Source: CAD feature listing. Evaluate the final solid. Frame: model axes, mm. A direction names the side the tool comes from. Give positions to 0.01 mm unless a question says otherwise; leave off trailing zeros. Answer as a JSON object with one key per item and string values. Group by question number.
Item 1: First-contact query: pin 1 Ø1.4 at (x, z) = (81.5, -1) entering from +Y (3 decimals); pin 2 Ø3.5 at (x, z) = (90.5, -1) entering from -Y; pin 3 Ø2.5 at (x, y) = (59.5, 0.5) entering from -Z (3 decimals). Flat tips, straight axial feed; report the tip coordinate or a pass-through.
Item 2: Ray query, probe 1 along Y at (x, z) = (92.5, -1) (3 decimals); probe 2 along Y at (x, z) = (48.5, -7.25) (3 decimals). Return the intervals inside material, ascending. Write a range as from..to.
Item 3: Pull-direction query (Z, two-part tool) for faces 5 (the face through (74, -7, 10)), 6 (the face through (74, 0, -3.365)), 7 (the face through (74, -8.5, -4)); classes: pulls with the +Z half, pulls with the -Z half, needs draft (parallel to the pull), parting line crosses it, or undercut.
Item 4: Access query for faces 1 (the face through (73.95, -4.18, -5.24)), 2 (the face through (74, -3.365, 0)), 3 (the face through (74, 0, 3.365)), 4 (the face through (74, 10, -7)). Directions: +Z, -Z, +X, -X, +Y, -Y. A direction counts if a zero-diameter tool reaches every point of the face in a straight line with its end or side. Return the directions, or none.
from build123d import *

# Parameters (mm, degrees)
BOSS_EXTRUDE1_DEPTH = 150


with BuildPart() as part:
    # Sketch1 → Boss-Extrude1 (new body)
    with BuildSketch(Plane(origin=(0, 0, 0), x_dir=(0, 0, -1), z_dir=(1, 0, 0))):
        Polygon((8.939339828, -10), (5.995, -7.055660172), (5.995, -8.5), (2.63, -8.5), (4.13, -10), align=None)
        Polygon((8.5, -5.995), (7.055660172, -5.995), (10, -8.939339828), (10, -4.13), (8.5, -2.63), align=None)
        Polygon((7.055660172, -5.995), (3.365, -2.304339828), (3.365, -3.365), (2.304339828, -3.365), (5.995, -7.055660172), (8.939339828, -10), (10, -10), (10, -8.939339828), align=None)
        with BuildLine():
            Line((3.365, -3.365), (3.365, -2.304339828))
            Line((3.365, -2.304339828), (2.216672281, -1.15601211))
            ThreePointArc((2.216672281, -1.15601211), (1.767766953, -1.767766953), (1.15601211, -2.216672281))
            Line((1.15601211, -2.216672281), (2.304339828, -3.365))
            Line((2.304339828, -3.365), (3.365, -3.365))
        make_face()
        with BuildLine():
            Line((3.365, -2.304339828), (3.365, 2.304339828))
            Line((3.365, 2.304339828), (2.216672281, 1.15601211))
            ThreePointArc((2.216672281, 1.15601211), (2.428135159, 0.595113139), (2.5, 0))
            ThreePointArc((2.5, 0), (2.428135159, -0.595113139), (2.216672281, -1.15601211))
            Line((2.216672281, -1.15601211), (3.365, -2.304339828))
        make_face()
        with BuildLine():
            Line((2.216672281, 1.15601211), (3.365, 2.304339828))
            Line((3.365, 2.304339828), (3.365, 3.365))
            Line((3.365, 3.365), (2.304339828, 3.365))
            Line((2.304339828, 3.365), (1.15601211, 2.216672281))
            ThreePointArc((1.15601211, 2.216672281), (1.767766953, 1.767766953), (2.216672281, 1.15601211))
        make_face()
        with BuildLine():
            ThreePointArc((-1.15601211, 2.216672281), (0, 2.5), (1.15601211, 2.216672281))
            Line((1.15601211, 2.216672281), (2.304339828, 3.365))
            Line((2.304339828, 3.365), (-2.304339828, 3.365))
            Line((-2.304339828, 3.365), (-1.15601211, 2.216672281))
        make_face()
        with BuildLine():
            ThreePointArc((-2.216672281, 1.15601211), (-1.767766953, 1.767766953), (-1.15601211, 2.216672281))
            Line((-1.15601211, 2.216672281), (-2.304339828, 3.365))
            Line((-2.304339828, 3.365), (-3.365, 3.365))
            Line((-3.365, 3.365), (-3.365, 2.304339828))
            Line((-3.365, 2.304339828), (-2.216672281, 1.15601211))
        make_face()
        with BuildLine():
            ThreePointArc((-2.216672281, -1.15601211), (-2.5, 0), (-2.216672281, 1.15601211))
            Line((-2.216672281, 1.15601211), (-3.365, 2.304339828))
            Line((-3.365, 2.304339828), (-3.365, -2.304339828))
            Line((-3.365, -2.304339828), (-2.216672281, -1.15601211))
        make_face()
        with BuildLine():
            Line((-2.304339828, -3.365), (-1.15601211, -2.216672281))
            ThreePointArc((-1.15601211, -2.216672281), (-1.767766953, -1.767766953), (-2.216672281, -1.15601211))
            Line((-2.216672281, -1.15601211), (-3.365, -2.304339828))
            Line((-3.365, -2.304339828), (-3.365, -3.365))
            Line((-3.365, -3.365), (-2.304339828, -3.365))
        make_face()
        with BuildLine():
            Line((-2.304339828, -3.365), (2.304339828, -3.365))
            Line((2.304339828, -3.365), (1.15601211, -2.216672281))
            ThreePointArc((1.15601211, -2.216672281), (0, -2.5), (-1.15601211, -2.216672281))
            Line((-1.15601211, -2.216672281), (-2.304339828, -3.365))
        make_face()
        Polygon((10, 4.13), (10, 8.939339828), (7.055660172, 5.995), (8.5, 5.995), (8.5, 2.63), align=None)
        Polygon((7.055660172, 5.995), (10, 8.939339828), (10, 10), (8.939339828, 10), (5.995, 7.055660172), (2.304339828, 3.365), (3.365, 3.365), (3.365, 2.304339828), align=None)
        Polygon((5.995, 7.055660172), (8.939339828, 10), (4.13, 10), (2.63, 8.5), (5.995, 8.5), align=None)
        Polygon((-8.939339828, 10), (-5.995, 7.055660172), (-5.995, 8.5), (-2.63, 8.5), (-4.13, 10), align=None)
        Polygon((-3.365, 3.365), (-2.304339828, 3.365), (-5.995, 7.055660172), (-8.939339828, 10), (-10, 10), (-10, 8.939339828), (-7.055660172, 5.995), (-3.365, 2.304339828), align=None)
        Polygon((-8.5, 5.995), (-7.055660172, 5.995), (-10, 8.939339828), (-10, 4.13), (-8.5, 2.63), align=None)
        Polygon((-10, -8.939339828), (-7.055660172, -5.995), (-8.5, -5.995), (-8.5, -2.63), (-10, -4.13), align=None)
        Polygon((-5.995, -7.055660172), (-2.304339828, -3.365), (-3.365, -3.365), (-3.365, -2.304339828), (-7.055660172, -5.995), (-10, -8.939339828), (-10, -10), (-8.939339828, -10), align=None)
        Polygon((-5.995, -8.5), (-5.995, -7.055660172), (-8.939339828, -10), (-4.13, -10), (-2.63, -8.5), align=None)
    extrude(amount=BOSS_EXTRUDE1_DEPTH)


solid = part.part
Worked answers:
{
 "1": {"pin 1": "y = 3.365", "pin 2": "y = -8.62", "pin 3": "z = -3.365"},
 "2": {"probe 1": "-3.365..-2.291, 2.291..3.365", "probe 2": "-10..-5.995, 5.995..10"},
 "3": {"face 5": "pulls with the +Z half", "face 6": "pulls with the -Z half", "face 7": "undercut"},
 "4": {"face 1": "+X, -X", "face 2": "+X, -X, -Y", "face 3": "+Z, +X, -X", "face 4": "+Z, -Z, +X, -X, +Y"}
}
